Can you work these out from the model? Positions are in its coordinate system, mm. Face numbers are marked on the shaded views. A direction names the side the tool comes from. Give positions to 0.01 mm unless a question says otherwise; leave off trailing zeros. Loops run counter-clockwise (first coordinate to the right, second up) from the corner with the lowest first, then second, coordinate; pieces in that order, holes last. Notation, with made-up numbers: (30, -21) - (70, -21) arc R12 cw to (70, -2) - close; hole circle Ø11 at (70, 42.25). An arc over 180 degrees is marked (long way). Answer in a Markdown table with one row per item.
Autodesk Fusion 360 part; units mm, degrees
sketch "Sketch2" plane through (0, 0, 0) normal (0, -1, 0) x (1, 0, 0)
  circle A0 centre (0, 0) radius 0.9974
  circle A1 centre (0, 0) radius 2.2479
extrude "Extrude1" add sketch "Sketch2" along normal blind 7.25 contours A0
extrude "Extrude2" add 1 faces at (-0.2437, -7.25, 0.2261) along direction (0, -1, 0) blind 7.366
extrude "Extrude4" cut 1 faces at (-0.2437, -14.616, 0.2261) along direction (0, 1, 0) blind 2.54
sketch "Sketch3" plane through (0, 0, 0) normal (0, 1, 0) x (-1, 0, 0)
  circle A0 centre (0, 0) radius 0.9974
  circle A1 centre (0, 0) radius 2.2479
  dimension "d14" = 4.4958
extrude "Extrude5" add sketch "Sketch3" along normal blind 3.81 contours A0 | A1
extrude "Extrude6" add 1 faces at (-1.819, 0, -0.1612) along direction (0, -1, 0) blind 1.016
extrude "Extrude7" cut 1 faces at (-0.7569, 3.81, -0.3251) along direction (0, -1, 0) blind 1.27
fillet "Fillet1" radius 1.016 1 edges at (2.0958, 2.54, 0.8129)
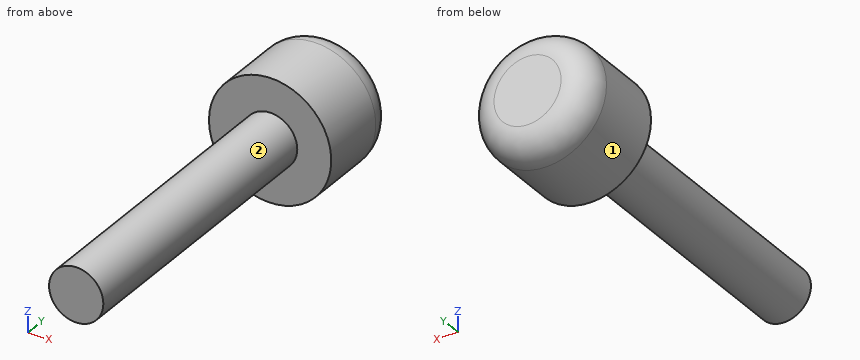
Q1. Imagine slicing it at A-A, the plane z = 0. Write out the boundary of the cut face in (x, y).
Checked values:
| item | result |
|---|---|
| outline | (-2.25, -1.02) - (-1, -1.02) - (-1, -12.08) - (1, -12.08) - (1, -1.02) - (2.25, -1.02) - (2.25, 1.52) arc R1.02 ccw to (1.23, 2.54) - (-1.23, 2.54) arc R1.02 ccw to (-2.25, 1.52) - close |
Q2. Imagine slicing it at B-B, the plane x = 0. Write out the boundary of the cut face in (y, z), and give its area (3 significant figures).
Checked values:
| item | result |
|---|---|
| outline | (-12.08, -1) - (-1.02, -1) - (-1.02, -2.25) - (1.52, -2.25) arc R1.02 ccw to (2.54, -1.23) - (2.54, 1.23) arc R1.02 ccw to (1.52, 2.25) - (-1.02, 2.25) - (-1.02, 1) - (-12.08, 1) - close |
| area | 37.6 mm² |
Q3. Imagine slicing it at C-C, the plane y = -1.25. Write out the boundary of the cut face in (x, z), and give its area (3 significant figures).
Checked values:
| item | result |
|---|---|
| outline | circle Ø1.99 at (0, 0) |
| area | 3.13 mm² |
Q4. If I drill on line 1 (Y direction, x = -1.25, z = 0); line 2 (Z direction, x = 1.2, y = 0.5); line 3 (X direction, y = -2.75, z = 0.5), over which ranges is the centre line in solid material (lowest first)? Write a range as [from, to].
Checked values:
| item | result |
|---|---|
| line 1 | y = [-1.02, 2.54] |
| line 2 | z = [-1.9, 1.9] |
| line 3 | x = [-0.86, 0.86] |
Q5. On a 3-axis mill with a long thin cutter (end or side, diameter ignored), from which of +Z, -Z, +X, -X, +Y, -Y can I reach the whole of each face in a straight line? I mean the marked faces 1 and 2. Say none if no direction works.
Checked values:
| item | result |
|---|---|
| face 1 | +Y, -Y |
| face 2 | -Y |
Q6. For pin 1 (1.5 mm diameter, centred on x = 1, y = -6.5, fed in from -Z), with a flat end and sliding along its axis, tell me the tip position at first contact or that it passes through.
Checked values:
| item | result |
|---|---|
| pin 1 | stops at z = -0.97 |
